Could you check a few things on this drawing? It's one solid part, dimensions in mm from its lowest x, y, z. Round coordinates to 2 decimals unless told otherwise and drop trailing zeros. Write each loop counter-clockwise with the first axis right and the second up, starting at its lowest first coordinate (ties: lowest second). Pieces come first, ordered by that corner, then holes. Notation, with made-up numbers: M -12.5,60 L 26.5,60 A15 ccw 26.5,80 Z; hole C 72,56.25 d1. An arc over 180 degrees is marked long. One line per question, with ' | ' between items. Start each with the question number.
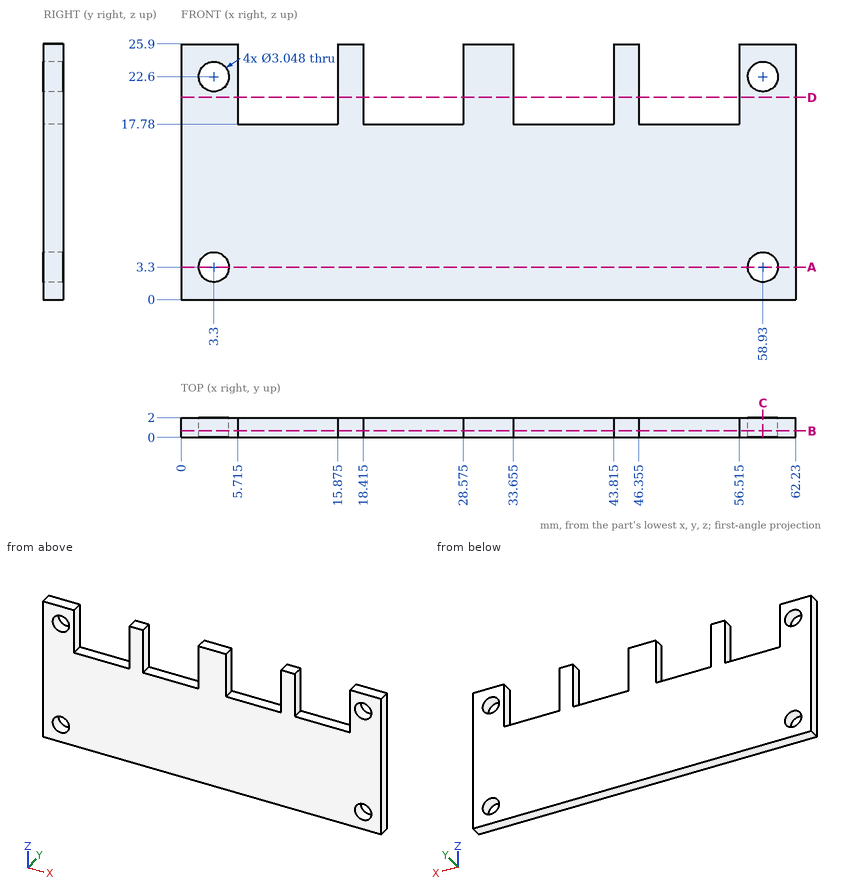
1. Suppose I cut it at D-D (z = 20.5). Write out the boundary of the cut face in (x, y) (3 decimals), and give its area (3 significant figures).
2. Suppose I cut it at B-B (y = 0.65). Write out the boundary of the cut face in (x, z) (3 decimals).
3. Suppose I cut it at A-A (z = 3.3). Write out the boundary of the cut face in (x, y).
4. I'm going to push a flat-ended pin straight in: P1, Ø0.6, axis at x = 11, y = 0.5, coming from the +Z side. Where does the tip first touch, or does it pass through?
5. I need wall thicknesses on line 1 along X through (y, z) = (0.85, 3.3); line 2 along X through (y, z) = (0.5, 24.5) (3 decimals); line 3 along Z through (x, y) = (4, 0.7). Which ranges of each line are inside material? Lowest first, please. Write a range as from..to.
6. Suppose I cut it at C-C (x = 58.93). Write out the boundary of the cut face in (y, z).
Computed:
1) outline: M 0,0 L 5.715,0 L 5.715,2 L 0,2 Z; M 15.875,0 L 18.415,0 L 18.415,2 L 15.875,2 Z; M 28.575,0 L 33.655,0 L 33.655,2 L 28.575,2 Z; M 43.815,0 L 46.355,0 L 46.355,2 L 43.815,2 Z; M 56.515,0 L 62.23,0 L 62.23,2 L 56.515,2 Z | area: 43.2 mm²
2) outline: M 0,0 L 62.23,0 L 62.23,25.9 L 56.515,25.9 L 56.515,17.78 L 46.355,17.78 L 46.355,25.9 L 43.815,25.9 L 43.815,17.78 L 33.655,17.78 L 33.655,25.9 L 28.575,25.9 L 28.575,17.78 L 18.415,17.78 L 18.415,25.9 L 15.875,25.9 L 15.875,17.78 L 5.715,17.78 L 5.715,25.9 L 0,25.9 Z; hole C 3.3,3.3 d3.048; hole C 3.3,22.6 d3.048; hole C 58.93,3.3 d3.048; hole C 58.93,22.6 d3.048
3) outline: M 0,0 L 1.78,0 L 1.78,2 L 0,2 Z; M 4.82,0 L 57.41,0 L 57.41,2 L 4.82,2 Z; M 60.45,0 L 62.23,0 L 62.23,2 L 60.45,2 Z
4) P1: stops at z = 17.78
5) line 1: x = 0..1.78, 4.82..57.41, 60.45..62.23 | line 2: x = 0..5.715, 15.875..18.415, 28.575..33.655, 43.815..46.355, 56.515..62.23 | line 3: z = 0..1.95, 4.65..21.25, 23.95..25.9
6) outline: M 0,0 L 2,0 L 2,1.78 L 0,1.78 Z; M 0,4.82 L 2,4.82 L 2,21.08 L 0,21.08 Z; M 0,24.12 L 2,24.12 L 2,25.9 L 0,25.9 Z
